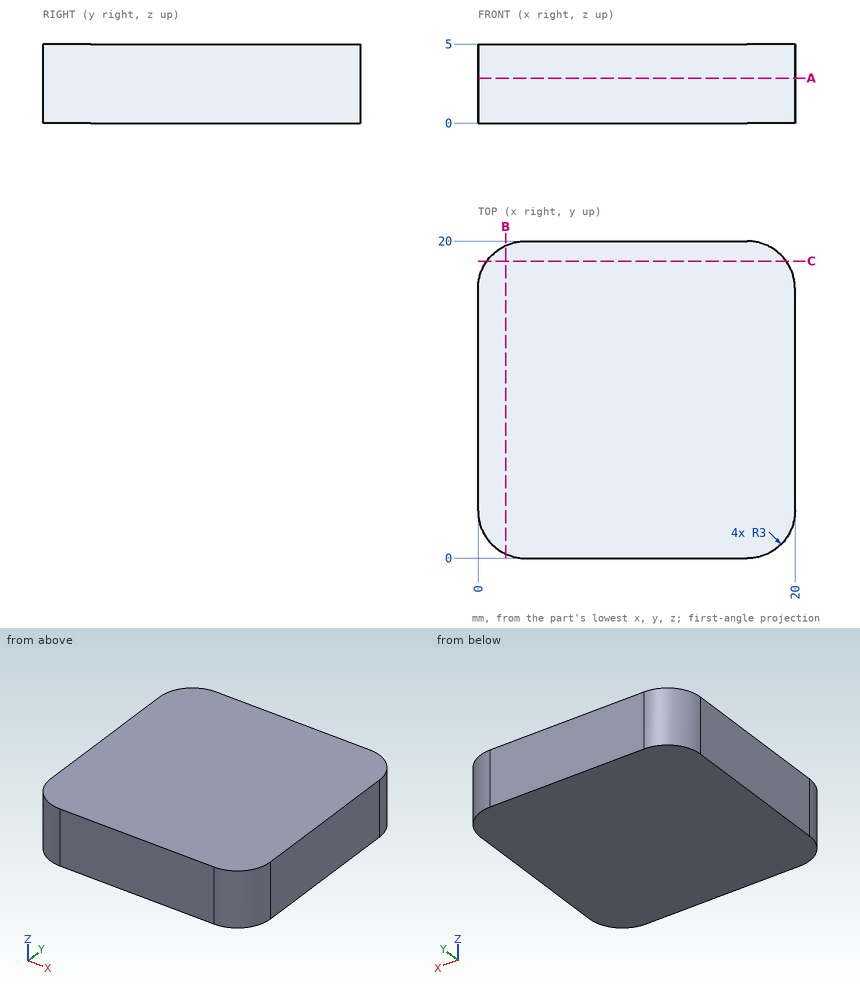
Study the drawing (mm; zero at the part's minimum x, y, z) and answer. Coordinates: 2 decimals unless noted, no trailing zeros. Write each loop counter-clockwise with the first axis right and the second up, starting at its lowest first coordinate (ties: lowest second). Pieces come first, ordered by that corner, then holes. Notation, with made-up numbers: M -22.75,56 L -7.75,56 A19 cw -7.75,69 Z; hole C -39,41 d8. An arc over 180 degrees is marked long. Use one line per item in the form item = value.
Item 1: Find section B-B, the plane x = 1.75. Give the vertices of the cut face in (y, z), plus the area to 3 significant figures.
Model answer:
outline = M 0.27,0 L 19.73,0 L 19.73,5 L 0.27,5 Z
area = 97.3 mm2
Item 2: Find the intervals of material crossed by probe 1 along Y at (x, z) = (17.75, 2.6); probe 2 along X at (y, z) = (18.75, 4.65), in increasing order.
Model answer:
probe_1 = 0.1 to 19.9
probe_2 = 0.56 to 19.44
Item 3: Find section C-C, the plane y = 18.75. Give the vertices of the cut face in (x, z).
Model answer:
outline = M 0.56,0 L 19.44,0 L 19.44,5 L 0.56,5 Z
Item 4: Find section A-A, the plane z = 2.85. Give the vertices of the cut face in (x, y).
Model answer:
outline = M 0,3 A3 ccw 3,0 L 17,0 A3 ccw 20,3 L 20,17 A3 ccw 17,20 L 3,20 A3 ccw 0,17 Z
